from build123d import *

# Parameters (mm, degrees)
CROQUIS1_R                   = 30
CROQUIS1_R_2                 = 25
SALIENTE_EXTRUIR1_DEPTH      = 225
CROQUIS2_R                   = 42.5
SALIENTE_EXTRUIR2_DEPTH      = 5
TALADRO_DE_MARGEN_PARA_M31_D = 3.4


with BuildPart() as part:
    # Croquis1 → Saliente-Extruir1 (new, symmetric)
    with BuildSketch(Plane(origin=(0, 0, 0), x_dir=(1, 0, 0), z_dir=(0, 1, 0))):
        with Locations(Location((0, 0, 0), (0, 0, 270))):
            Circle(CROQUIS1_R)
        with Locations(Location((0, 0, 0), (0, 0, 270))):
            Circle(CROQUIS1_R_2, mode=Mode.SUBTRACT)
    extrude(amount=SALIENTE_EXTRUIR1_DEPTH, both=True)

    # Croquis2 → Saliente-Extruir2 (add)
    with BuildSketch(Plane(origin=(0, 225, 0), x_dir=(1, 0, 0), z_dir=(0, 1, 0))):
        with Locations(Location((0, 0, 0), (0, 0, 270))):
            Circle(CROQUIS2_R)
    saliente_extruir2 = extrude(amount=SALIENTE_EXTRUIR2_DEPTH)

    # Taladro de margen para M31 (through all)
    with Locations(Plane(origin=(0, 225, 0), x_dir=(-1, 0, 0), z_dir=(0, -1, 0))):
        with Locations((0, -35), (-24.748737342, -24.748737342), (-35, 0), (-24.748737342, 24.748737342), (0, 35), (24.748737342, 24.748737342), (35, 0), (24.748737342, -24.748737342)):
            taladro_de_margen_para_m31 = Hole(TALADRO_DE_MARGEN_PARA_M31_D / 2)

    # Simetría1: Saliente-Extruir2, Taladro de margen para M31 across plane
    add(saliente_extruir2.mirror(Plane.ZX))
    add(taladro_de_margen_para_m31.mirror(Plane.ZX), mode=Mode.SUBTRACT)


solid = part.part
The listing builds one solid part. Answer for the finished solid, in the listing's coordinates (mm). A direction names the side the tool comes from. Give positions to 0.01 mm unless a question says otherwise; leave off trailing zeros. Order: outer loops, then holes, each group sorted by start corner. A loop starts at its lowest first (then second) coordinate and runs counter-clockwise, first axis right, second up. Notation, with made-up numbers: (49.5, -14) - (89.5, -14) arc R26 cw to (89.5, 10) - close; hole circle Ø3 at (58.5, 20). An arc over 180 degrees is marked (long way). One line per item, written item: value. Start each with the question number.
1) A tool of negligible diameter and unlimited length cuts with its end or side. For faces 1 (the face through (-25.861, -227.465, -33.727)), 2 (the face through (0, 225, 0)), from which of +Z, -Z, +X, -X, +Y, -Y can it reach the whole face along a straight path? Write none if from no direction.
2) A cutting plane is placed at A-A on y = -51.5. Give the vertices of the cut face in (x, z), then the cut area to 3 significant figures.
3) The mould has two halves that part along Y. Classify faces 3 (the face through (1, 230, -1)), 4 (the face through (0, -225, 0)), 5 (the face through (1, -230, -1)): released by +Y, released by -Y, zero draft, split by the parting line, or undercut.
4) A cutting plane is placed at B-B on x = 12.5. Give the vertices of the cut face in (y, z).
5) Find the intervals of material crossed by L1, parallel to Y at x = -0.5, z = -13; L2, parallel to X at y = -5, z = -1.5, in increasing order.
6) Given pin 1 Ø4.5 at (x, z) = (0, -35) entering from +Y; pin 2 Ø8 at (x, y) = (28.5, -125.5) entering from +Z; pin 3 Ø5 at (y, z) = (65.5, -29) entering from +X; pin 4 Ø2.5 at (x, z) = (-35, 0) entering from -Y, each flat-ended and moving along its own axis, determine where each tip first touches the part or whether it passes through.
Answer sheet:
1. face 1: +Y, -Y
1. face 2: none
2. outline: circle Ø60 at (0, 0); hole circle Ø50 at (0, 0)
2. area: 864 mm2
3. face 3: released by +Y
3. face 4: undercut
3. face 5: released by -Y
4. outline: (-230, -40.62) - (-225, -40.62) - (-225, -27.27) - (225, -27.27) - (225, -40.62) - (230, -40.62) - (230, 40.62) - (225, 40.62) - (225, 27.27) - (-225, 27.27) - (-225, 40.62) - (-230, 40.62) - close; hole (-225, -21.65) - (225, -21.65) - (225, 21.65) - (-225, 21.65) - close
5. L1: y = -230 to -225, 225 to 230
5. L2: x = -29.96 to -24.95, 24.95 to 29.96
6. pin 1: stops at y = 230
6. pin 2: stops at z = 17.31
6. pin 3: stops at x = 14.06
6. pin 4: passes through
